Check sheet for the modelled part. Datum: model origin and axes. Units: mm. Give positions to 0.01 mm unless a question says otherwise; leave off trailing zeros. Loops run counter-clockwise (first coordinate to the right, second up) from the corner with the lowest first, then second, coordinate; pieces in that order, holes last. Notation, with made-up numbers: (21.5, 18) -> (63.5, 18) arc R29 ccw to (63.5, 56) -> close; hole circle Ø2 at (-28, -36.75). An arc over 180 degrees is marked (long way). Answer as CSV lines item,"result". Start each with the question number.
(1) Material ranges on line 1 (Y direction, x = -1, z = 0.05); line 2 (Y direction, x = 4.25, z = -0.05); line 3 (X direction, y = 4.25, z = 0), recorded low to high. Write a range as from..to.
(2) Section check D-D on x = -2. Enter the section's corners in (y, z) (3 decimals), plus the area to 3 significant figures.
(3) Section check A-A on y = 7.25. Enter the section's corners in (x, z) (3 decimals).
(4) Section check B-B on x = 3.5. State how many separate pieces and enclosed holes the cut face has, plus the area to 3 significant figures.
from build123d import *

# Parameters (mm, degrees)
FRAME_OUTLINE_W     = 1
FRAME_OUTLINE_H     = 0.115
FRAME_OUTLINE_W_2   = 0.1
FRAME_OUTLINE_H_2   = 1
BOSS_EXTRUDE1_DEPTH = 0.125
FILLET1_R           = 0.5
FILLET2_R           = 0.4
CUT_EXTRUDE1_DEPTH  = 12.518354917


with BuildPart() as part:
    # frame_outline → Boss-Extrude1 (new, symmetric)
    with BuildSketch(Plane.XY):
        Polygon((0.05, 0.3), (0.05, 1.5), (0.1, 1.5), (0.1, 2.562485241), (0.05, 2.562485241), (-0.008875073, 2.811860782), (0.203530984, 3.066347223), (0.655022448, 4.283241722), (0.625059951, 4.94163014), (-0.232915246, 5.208434363), (-1.213255559, 4.94163014), (-1.763721297, 4.6), (-4.5, 4.6), (-4.5, 10.6), (4.5, 10.6), (4.5, 4.6), (2.518192453, 0.35), (1.5, 0.35), (1.5, 0.05), (0.3, 0.05), (0.3, 0.3), align=None)
        with Locations((0, 8.1575)):
            Rectangle(FRAME_OUTLINE_W, FRAME_OUTLINE_H, mode=Mode.SUBTRACT)
        with Locations((-2.55, 7.6)):
            Rectangle(FRAME_OUTLINE_W_2, FRAME_OUTLINE_H_2, mode=Mode.SUBTRACT)
        with Locations((-2.55, 5.6)):
            Rectangle(FRAME_OUTLINE_W_2, FRAME_OUTLINE_H_2, mode=Mode.SUBTRACT)
        with Locations((2.55, 7.6)):
            Rectangle(FRAME_OUTLINE_W_2, FRAME_OUTLINE_H_2, mode=Mode.SUBTRACT)
        with Locations((2.55, 5.6)):
            Rectangle(FRAME_OUTLINE_W_2, FRAME_OUTLINE_H_2, mode=Mode.SUBTRACT)
        with Locations((2.55, 2.6)):
            Rectangle(FRAME_OUTLINE_W_2, FRAME_OUTLINE_H_2, mode=Mode.SUBTRACT)
        with Locations((-3.5, 8.1575)):
            Rectangle(FRAME_OUTLINE_W, FRAME_OUTLINE_H, mode=Mode.SUBTRACT)
        with Locations((3.5, 8.1575)):
            Rectangle(FRAME_OUTLINE_W, FRAME_OUTLINE_H, mode=Mode.SUBTRACT)
        with Locations((-3.5, 5.0425)):
            Rectangle(FRAME_OUTLINE_W, FRAME_OUTLINE_H, mode=Mode.SUBTRACT)
        with Locations((3.5, 5.0425)):
            Rectangle(FRAME_OUTLINE_W, FRAME_OUTLINE_H, mode=Mode.SUBTRACT)
    extrude(amount=BOSS_EXTRUDE1_DEPTH, both=True)

    # Fillet1
    # the kernel refuses this fillet: 0.5 mm, written as the material it adds along each edge
    with BuildSketch(Plane(origin=(1.5, 0.35, 0.125), x_dir=(0, -1, 0), z_dir=(0, 0, -1))) as fillet1_piece_1:
        with BuildLine():
            CenterArc((0.5, -0.458257569), FILLET1_R, 113.578178478, 66.421821522)
            Line((0, -0.458257569), (0, 0))
            Line((0, 0), (0.3, 0))
        make_face()
    extrude(amount=0.25)
    with BuildSketch(Plane(origin=(0.3, 0.3, -0.125), x_dir=(0, -1, 0), z_dir=(0, 0, 1))) as fillet1_piece_2:
        with BuildLine():
            CenterArc((0.455718914, -0.455718914), FILLET1_R, 114.295188945, 41.409622109)
            Line((0, -0.25), (0, 0))
            Line((0, 0), (0.25, 0))
        make_face()
    extrude(amount=0.25)

    # Fillet2
    fillet2_edges = [part.edges().sort_by_distance(p)[0] for p in [
        (-0.008875073, 2.811860782, 0),
        (0.203530984, 3.066347223, 0),
        (0.655022448, 4.283241722, 0),
        (0.625059951, 4.94163014, 0),
        (-0.232915246, 5.208434363, 0),
        (-1.213255559, 4.94163014, 0),
        (-1.763721297, 4.6, 0),
    ]]
    fillet(fillet2_edges, radius=FILLET2_R)

    # Sketch1 → Cut-Extrude1 (cut, through all)
    with BuildSketch(Plane.XY.offset(0.125)):
        with BuildLine():
            Line((-4.5, 9.6), (-4.5, 10.6))
            Line((-4.5, 10.6), (-2.6, 10.6))
            ThreePointArc((-2.6, 10.6), (-3.313845854, 9.868537952), (-4.3, 9.6))
            Line((-4.3, 9.6), (-4.5, 9.6))
        make_face()
        with BuildLine():
            Line((4.5, 10.6), (4.5, 9.6))
            Line((4.5, 9.6), (4.3, 9.6))
            ThreePointArc((4.3, 9.6), (3.313845854, 9.868537952), (2.6, 10.6))
            Line((2.6, 10.6), (4.5, 10.6))
        make_face()
    extrude(amount=-CUT_EXTRUDE1_DEPTH, mode=Mode.SUBTRACT)


solid = part.part
Working result:
1,line 1,"y = 5..10.6"
1,line 2,"y = 4.06..9.6"
1,line 3,"x = 0.64..4.34"
2,outline,"(4.6, -0.125) -> (10.6, -0.125) -> (10.6, 0.125) -> (4.6, 0.125) -> close"
2,area,"1.50 mm^2"
3,outline,"(-4.5, -0.125) -> (-2.6, -0.125) -> (-2.6, 0.125) -> (-4.5, 0.125) -> close; (-2.5, -0.125) -> (2.5, -0.125) -> (2.5, 0.125) -> (-2.5, 0.125) -> close; (2.6, -0.125) -> (4.5, -0.125) -> (4.5, 0.125) -> (2.6, 0.125) -> close"
4,separate pieces,"3"
4,enclosed holes,"0"
4,area,"1.77 mm^2"
